from build123d import *

# Parameters (mm, degrees)
EXTRUSION1_DEPTH = 50
EXTRUSION2_REACH = 3
ESQUISSE2_R      = 1.5
EXTRUSION3_REACH = 3
ESQUISSE3_R      = 1.5


with BuildPart() as part:
    # Esquisse1 → Extrusion1 (new body)
    with BuildSketch(Plane(origin=(0, 0, 0), x_dir=(1, 0, 0), z_dir=(0, 1, 0))):
        Polygon((0, 0), (0, 21), (1, 21), (1, 1), (21, 1), (21, 0), align=None)
    extrude(amount=EXTRUSION1_DEPTH)

    # Esquisse2 → Extrusion2 (cut, up to next)
    with BuildSketch(Plane(origin=(1, 0, 0), x_dir=(0, 0, -1), z_dir=(1, 0, 0)), mode=Mode.PRIVATE) as extrusion2_sk1:
        with Locations((11, 6.5)):
            Circle(ESQUISSE2_R)
    extrusion2_tool1 = extrude(extrusion2_sk1.sketch, amount=-EXTRUSION2_REACH, mode=Mode.PRIVATE) & part.part
    add(extrusion2_tool1.solids().sort_by_distance((1, 6.5, -11))[0], mode=Mode.SUBTRACT)
    # Esquisse2 → Extrusion2 (cut, up to next)
    with BuildSketch(Plane(origin=(1, 0, 0), x_dir=(0, 0, -1), z_dir=(1, 0, 0)), mode=Mode.PRIVATE) as extrusion2_sk2:
        with Locations((11, 43.5)):
            Circle(ESQUISSE2_R)
    extrusion2_tool2 = extrude(extrusion2_sk2.sketch, amount=-EXTRUSION2_REACH, mode=Mode.PRIVATE) & part.part
    add(extrusion2_tool2.solids().sort_by_distance((1, 43.5, -11))[0], mode=Mode.SUBTRACT)

    # Esquisse3 → Extrusion3 (cut, up to next)
    with BuildSketch(Plane(origin=(0, 0, -1), x_dir=(-1, 0, 0), z_dir=(0, 0, -1)), mode=Mode.PRIVATE) as extrusion3_sk1:
        with Locations((-11, 43.5)):
            Circle(ESQUISSE3_R)
    extrusion3_tool1 = extrude(extrusion3_sk1.sketch, amount=-EXTRUSION3_REACH, mode=Mode.PRIVATE) & part.part
    add(extrusion3_tool1.solids().sort_by_distance((11, 43.5, -1))[0], mode=Mode.SUBTRACT)
    # Esquisse3 → Extrusion3 (cut, up to next)
    with BuildSketch(Plane(origin=(0, 0, -1), x_dir=(-1, 0, 0), z_dir=(0, 0, -1)), mode=Mode.PRIVATE) as extrusion3_sk2:
        with Locations((-11, 6.5)):
            Circle(ESQUISSE3_R)
    extrusion3_tool2 = extrude(extrusion3_sk2.sketch, amount=-EXTRUSION3_REACH, mode=Mode.PRIVATE) & part.part
    add(extrusion3_tool2.solids().sort_by_distance((11, 6.5, -1))[0], mode=Mode.SUBTRACT)


solid = part.part
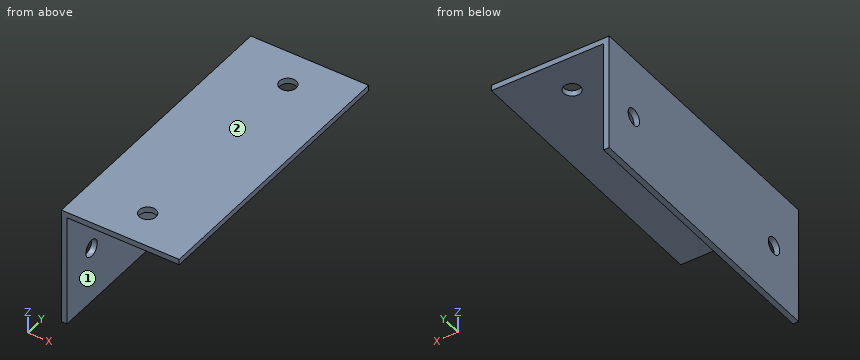
Source: CAD feature listing. Evaluate the final solid. Frame: model axes, mm. Face numbers are marked on the shaded views. A direction names the side the tool comes from. Coordinates: 2 decimals unless noted, no trailing zeros. Loops run counter-clockwise (first coordinate to the right, second up) from the corner with the lowest first, then second, coordinate; pieces in that order, holes last. Notation, with made-up numbers: M 40,78.5 L 90,78.5 A19 ccw 90,105.5 Z; hole C 54.25,-13 d10. An arc over 180 degrees is marked long. Answer in a Markdown table with one row per item.
Q1. Ray query, probe 1 along Y at (x, z) = (0.5, -11); probe 2 along X at (y, z) = (14, -2.25); probe 3 along Z at (x, y) = (1.75, 45). Return the intervals inside material, ascending. Write a range as from..to.
Answers below:
| item | result |
|---|---|
| probe 1 | y = 0..5, 8..42, 45..50 |
| probe 2 | x = 0..1 |
| probe 3 | z = -1..0 |
Q2. First-contact query: pin 1 (2 mm diameter, centred on y = 35.5, z = -14, fed in from +X); pin 2 (4 mm diameter, centred on x = 11, y = 43.5, fed in from -Z); pin 3 (2.5 mm diameter, centred on y = 43.5, z = -11, fed in from +X). Flat tips, straight axial feed; report the tip coordinate or a pass-through.
Answers below:
| item | result |
|---|---|
| pin 1 | stops at x = 1 |
| pin 2 | stops at z = -1 |
| pin 3 | passes through |
Q3. Section B-B on x = 11. Return the cut outline in (y, z), plus the area to 3 significant figures.
Answers below:
| item | result |
|---|---|
| outline | M 0,-1 L 5,-1 L 5,0 L 0,0 Z; M 8,-1 L 42,-1 L 42,0 L 8,0 Z; M 45,-1 L 50,-1 L 50,0 L 45,0 Z |
| area | 44.0 mm^2 |
Q4. Section C-C on y = 6.5. Return the cut outline in (x, z).
Answers below:
| item | result |
|---|---|
| outline | M 0,-21 L 1,-21 L 1,-12.5 L 0,-12.5 Z; M 0,-9.5 L 1,-9.5 L 1,-1 L 9.5,-1 L 9.5,0 L 0,0 Z; M 12.5,-1 L 21,-1 L 21,0 L 12.5,0 Z |
Q5. Set-up query: the marked faces 1 and 2. Return all of +Z, -Z, +X, -X, +Y, -Y with unobstructed straight access to the full face (end or side cutting, diameter ignored); none if empty.
Answers below:
| item | result |
|---|---|
| face 1 | -Z, +X, +Y, -Y |
| face 2 | +Z, +X, -X, +Y, -Y |
Q6. Section A-A on z = -11. Return the cut outline in (x, y), plus the area to 3 significant figures.
Answers below:
| item | result |
|---|---|
| outline | M 0,0 L 1,0 L 1,5 L 0,5 Z; M 0,8 L 1,8 L 1,42 L 0,42 Z; M 0,45 L 1,45 L 1,50 L 0,50 Z |
| area | 44.0 mm^2 |
Q7. Section D-D on y = 46.5. Return the cut outline in (x, z), plus the area to 3 significant figures.
Answers below:
| item | result |
|---|---|
| outline | M 0,-21 L 1,-21 L 1,-1 L 21,-1 L 21,0 L 0,0 Z |
| area | 41.0 mm^2 |
